Here's how the part is built. I have some questions about the finished solid (model axes, mm). Round coordinates to 2 decimals unless told otherwise and drop trailing zeros. Order: outer loops, then holes, each group sorted by start corner. A loop starts at its lowest first (then second) coordinate and runs counter-clockwise, first axis right, second up. Notation, with made-up numbers: M 24,7 L 61,7 A19 cw 61,15 Z; hole C -6.75,21.5 d11. An arc over 180 degrees is marked long. Use one line per item in the form item = value. Start each with the question number.
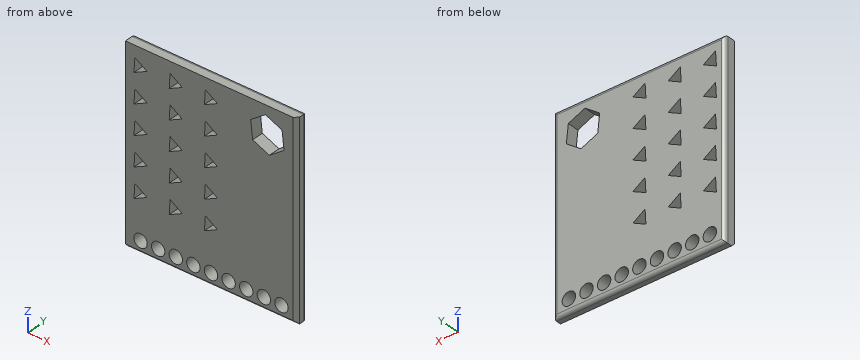
```python
from build123d import *

# Parameters (mm, degrees)
SKETCH1_W            = 145.774647888
SKETCH1_H            = 164.084507042
BOSS_EXTRUDE1_DEPTH  = 10
FILLET1_R            = 3
SKETCH2_R            = 5.718299624
CUT_EXTRUDE1_DEPTH   = 10
LPATTERN1_COUNT      = 9
LPATTERN1_PITCH      = 15
CUT_EXTRUDE2_DEPTH   = 10
LPATTERN2_COUNT      = 5
LPATTERN2_PITCH      = 25
LPATTERN2_COUNT_DIR2 = 3
LPATTERN2_PITCH_DIR2 = 30
CHAMFER1_SIZE        = 3


with BuildPart() as part:
    # Sketch1 → Boss-Extrude1 (new body)
    with BuildSketch(Plane(origin=(0, 0, 0), x_dir=(1, 0, 0), z_dir=(0, 1, 0))):
        Rectangle(SKETCH1_W, SKETCH1_H)
        Polygon((60.399278767, -67.985661607), (62.095878149, -52.558568526), (49.583923326, -43.375723821), (35.375369121, -49.619972196), (33.678769738, -65.047065276), (46.190724561, -74.229909982), align=None, mode=Mode.SUBTRACT)
    extrude(amount=BOSS_EXTRUDE1_DEPTH)

    # Fillet1
    fillet1_edges = [part.edges().sort_by_distance(p)[0] for p in [
        (-72.887323944, 10, 0),
        (0, 10, 82.042253521),
        (72.887323944, 10, 0),
        (0, 10, -82.042253521),
    ]]
    fillet(fillet1_edges, radius=FILLET1_R)

    # Sketch2 → Cut-Extrude1 (cut)
    with BuildSketch(Plane(origin=(0, 10, 0), x_dir=(1, 0, 0), z_dir=(0, 1, 0))):
        with Locations((-60.091318796, 71.08363321)):
            Circle(SKETCH2_R)
    cut_extrude1 = extrude(amount=-CUT_EXTRUDE1_DEPTH, mode=Mode.SUBTRACT)

    # LPattern1: Cut-Extrude1 ×9
    with Locations(*[(i * LPATTERN1_PITCH, 0, 0) for i in range(1, LPATTERN1_COUNT)]):
        add(cut_extrude1, mode=Mode.SUBTRACT)

    # Sketch3 → Cut-Extrude2 (cut)
    with BuildSketch(Plane(origin=(0, 10, 0), x_dir=(1, 0, 0), z_dir=(0, 1, 0))):
        Polygon((-64.940245829, 27.550407321), (-54.604744837, 34.374463584), (-65.682301413, 39.913241872), align=None)
    cut_extrude2 = extrude(amount=-CUT_EXTRUDE2_DEPTH, mode=Mode.SUBTRACT)

    # LPattern2: Cut-Extrude2 5 × 3
    with Locations(*[(j * LPATTERN2_PITCH_DIR2, 0, i * LPATTERN2_PITCH) for i in range(LPATTERN2_COUNT) for j in range(LPATTERN2_COUNT_DIR2) if (i, j) != (0, 0)]):
        add(cut_extrude2, mode=Mode.SUBTRACT)

    # Chamfer1
    chamfer1_edges = [part.edges().sort_by_distance(p)[0] for p in [
        (0, 0, -82.042253521),
        (72.887323944, 0, 0),
    ]]
    chamfer(chamfer1_edges, length=CHAMFER1_SIZE)


solid = part.part
```
1) If we section it at C-C on y = 1.5: Give the number of separate pieces and of enclosed holes in the cut face, then the cut area to 3 significant figures.
2) If we section it at B-B on x = 31: Write out the boundary of the cut face in (y, z), then the cut area to 3 significant figures.
3) If we section it at A-A on x = 58: Write out the boundary of the cut face in (y, z).
4) If I drill on line 1 (X direction, y = 1.25, z = 18.5); line 2 (Z direction, x = 42, y = 5.75); line 3 (X direction, y = 8.5, z = -3.5), over which ranges is the centre line in solid material (lowest first)?
5) Will this pin go through, and if not, where does the flat tip stop? pin 1 Ø9 at (x, z) = (59.91, -71.08) entering from -Y.
Completed:
q1.separate_pieces = 1
q1.enclosed_holes = 25
q1.area = 20,900 mm²
q2.outline = M 0,-79.04 L 3,-82.04 L 7,-82.04 A3 ccw 10,-79.04 L 10,-76.7 L 0,-76.7 Z; M 0,-65.47 L 10,-65.47 L 10,79.04 A3 ccw 7,82.04 L 0,82.04 Z
q2.area = 1,520 mm²
q3.outline = M 0,-79.04 L 3,-82.04 L 7,-82.04 A3 ccw 10,-79.04 L 10,-76.47 L 0,-76.47 Z; M 0,-65.69 L 10,-65.69 L 10,49.55 L 0,49.55 Z; M 0,69.04 L 10,69.04 L 10,79.04 A3 ccw 7,82.04 L 0,82.04 Z
q4.line_1 = -72.89 to -65.18, -58.96 to -35.18, -28.96 to -5.18, 1.04 to 71.14
q4.line_2 = -82.04 to -76.01, -66.16 to 46.71, 71.15 to 82.04
q4.line_3 = -72.49 to -65, -63.5 to -35, -33.5 to -5, -3.5 to 72.49
q5.pin_1 = through
